from build123d import *
from build123d.topology import SkipClean

# Parameters (mm, degrees)
SKETCH1_R           = 10
BOSS_EXTRUDE1_DEPTH = 45
FILLET1_R           = 5
SKETCH2_R           = 4
BOSS_EXTRUDE2_DEPTH = 162
SKETCH3_R           = 6
BOSS_EXTRUDE3_DEPTH = 2
BOSS_EXTRUDE4_DEPTH = 2.5
SKETCH5_OUTSIDE_W   = 64.776
SKETCH5_OUTSIDE_H   = 64.776
SKETCH5_OUTSIDE_R   = 6
CUT_EXTRUDE2_DEPTH  = 5
FILLET2_R           = 10
FILLET3_R           = 1


with BuildPart() as part:
    # Sketch1 → Boss-Extrude1 (new body)
    with BuildSketch(Plane(origin=(0, 0, 0), x_dir=(1, 0, 0), z_dir=(0, 1, 0))):
        with Locations(Location((0, 0, 0), (0, 0, 90))):
            Circle(SKETCH1_R)
    extrude(amount=BOSS_EXTRUDE1_DEPTH)

    # Fillet1
    fillet1_edges = [part.edges().sort_by_distance(p)[0] for p in [
        (0, 0, 10),
    ]]
    fillet(fillet1_edges, radius=FILLET1_R)

    # Sketch2 → Boss-Extrude2 (add)
    with BuildSketch(Plane(origin=(0, 45, 0), x_dir=(1, 0, 0), z_dir=(0, 1, 0))):
        with Locations(Location((0, 0, 0), (0, 0, 270))):
            Circle(SKETCH2_R)
    extrude(amount=BOSS_EXTRUDE2_DEPTH)

    # Sketch3 → Boss-Extrude3 (add)
    with BuildSketch(Plane(origin=(0, 207, 0), x_dir=(1, 0, 0), z_dir=(0, 1, 0))):
        with Locations(Location((0, 0, 0), (0, 0, 270))):
            Circle(SKETCH3_R)
    extrude(amount=BOSS_EXTRUDE3_DEPTH)

    # Sketch4 → Boss-Extrude4 (add, symmetric)
    with BuildSketch(Plane.XY):
        with BuildLine():
            Line((-6, 209), (6, 209))
            ThreePointArc((6, 209), (0, 212), (-6, 209))
        make_face()
    extrude(amount=BOSS_EXTRUDE4_DEPTH, both=True)

    # Sketch5 outside → Cut-Extrude2 (cut)
    with SkipClean():  # the faces are left unmerged after this step: merging them gives an invalid solid
        with BuildSketch(Plane.XZ.offset(-207)):
            Rectangle(SKETCH5_OUTSIDE_W, SKETCH5_OUTSIDE_H)
            with Locations(Location((0, 0, 0), (0, 0, 204.624318352))):
                Circle(SKETCH5_OUTSIDE_R, mode=Mode.SUBTRACT)
        extrude(amount=-CUT_EXTRUDE2_DEPTH, mode=Mode.SUBTRACT)
    add(part.part.scale(1), mode=Mode.REPLACE)  # the faces are merged on a copy

    # Fillet2
    # the kernel refuses this fillet: 10 mm, written as the material it adds along each edge
    with BuildSketch(Plane(origin=(0, 45, 0), x_dir=(0, 0, 1), z_dir=(-1, 0, 0))) as fillet2_piece_1:
        with BuildLine():
            CenterArc((14, 9.16515139), FILLET2_R, 180, 66.421821522)
            Line((10, 0), (9.92, -0.183303028))
            ThreePointArc((9.92, -0.183303028), (7, -0.2), (4, -0.2))
            Line((4, -0.2), (3.8, 0))
            Line((3.8, 0), (3.8, 9.16515139))
            Line((3.8, 9.16515139), (4, 9.16515139))
        make_face()
    revolve(axis=Axis((0, 45, 0), (0, 1, 0)))

    # Fillet3
    # the kernel refuses this fillet: 1 mm, written as the material it takes off along each edge
    with BuildSketch(Plane(origin=(0, 204.5, -2.5), x_dir=(0.9118550245849949, 0.41051238000710544, 0), z_dir=(0.41051238000710544, -0.9118550245849949, 0))) as fillet3_piece_1_section:
        with BuildLine():
            CenterArc((7.5 - FILLET3_R, FILLET3_R), FILLET3_R, 270, 90)
            Line((7.5, FILLET3_R), (7.5, 0))
            Line((7.5, 0), (7.5 - FILLET3_R, 0))
        make_face()
    fillet3_piece_1 = revolve(axis=Axis((0, 204.5, -2.5), (0, 0, 1)), revolution_arc=131.52594845, mode=Mode.PRIVATE)
    fillet3_piece_1 = split(fillet3_piece_1, bisect_by=Plane(origin=(0, 209, -2.216936938), z_dir=(0, 1, 0)), keep=Keep.TOP, mode=Mode.PRIVATE)
    add(fillet3_piece_1, mode=Mode.SUBTRACT)
    with BuildSketch(Plane(origin=(0, 204.5, 2.5), x_dir=(0.9118550245849949, 0.4105123800071055, 0), z_dir=(0.4105123800071055, -0.9118550245849949, 0))) as fillet3_piece_2_section:
        with BuildLine():
            CenterArc((7.5 - FILLET3_R, -FILLET3_R), FILLET3_R, 0, 90)
            Line((7.5 - FILLET3_R, 0), (7.5, 0))
            Line((7.5, 0), (7.5, -FILLET3_R))
        make_face()
    fillet3_piece_2 = revolve(axis=Axis((0, 204.5, 2.5), (0, 0, 1)), revolution_arc=131.52594845, mode=Mode.PRIVATE)
    fillet3_piece_2 = split(fillet3_piece_2, bisect_by=Plane(origin=(0, 209, 2.216936937), z_dir=(0, 1, 0)), keep=Keep.TOP, mode=Mode.PRIVATE)
    add(fillet3_piece_2, mode=Mode.SUBTRACT)


solid = part.part
Design review of the part built by this model. Coordinates are the model's own, in mm. Give positions to 0.01 mm unless a question says otherwise; leave off trailing zeros. Loops run counter-clockwise (first coordinate to the right, second up) from the corner with the lowest first, then second, coordinate; pieces in that order, holes last. Notation, with made-up numbers: (29, 79) - (68, 79) arc R18 cw to (68, 102) - close; hole circle Ø1 at (78.25, -30). An arc over 180 degrees is marked (long way). Use CSV: the item, a comma, the result in double quotes. Start each with the question number.
1. Insertion check: P1, Ø12, axis at x = 1, y = 80, coming from the -Z side; P2, Ø1, axis at x = 0.5, z = -3.5, coming from the +Y side; P3, Ø1.6, axis at x = 2, y = 209.5, coming from the +Z side. Each pin has a flat end and moves straight along its axis. Give the tip position at first contact, or say it passes through.
2. Wall thickness on L1, parallel to X at y = 124, z = 0.5; L2, parallel to Z at x = -0.25, y = 39; L3, parallel to Y at x = 1.5, z = 4.5: over which ranges is each line inside the solid? List them lowest first.
3. Draft analysis for pull direction Y (two halves, no side actions). For faces 1 (the flat face through (-3.92, 207, -1.42)), 2 (the cylindrical face through (9.76, 24.72, 2.17)), 3 (the flat face through (0, 0, 0)), state which applies: released by +Y, released by -Y, zero draft, split by the parting line, or undercut.
4. Add section A-A (y = 127). State the section outline as (x, z) points, plus the area to 3 significant figures.
Results found:
1,P1,"stops at z = -4"
1,P2,"stops at y = 209"
1,P3,"stops at z = 5.84"
2,L1,"x = -3.97 to 3.97"
2,L2,"z = -10 to 10"
2,L3,"y = 0 to 50.38, 207 to 209"
3,face 1,"undercut"
3,face 2,"zero draft"
3,face 3,"released by -Y"
4,outline,"circle Ø8 at (0, 0)"
4,area,"50.3 mm²"
